Could you check a few things on this drawing? It's one solid part, dimensions in mm from its lowest x, y, z. Give positions to 0.01 mm unless a question says otherwise; leave off trailing zeros. Order: outer loops, then holes, each group sorted by start corner. A loop starts at its lowest first (then second) coordinate and runs counter-clockwise, first axis right, second up. Notation, with made-up numbers: (38.25, -13) -> (84.25, -13) arc R25 cw to (84.25, 2) -> close; hole circle Ø9 at (34, 18). An arc over 180 degrees is marked (long way). Write each question's results on one line, items separated by ' | '. Start each with the question number.
Q1. I'm going to push flat-ended pins straight in: pin 1 (1.5 mm diameter, centred on x = 97, z = 1.5, fed in from -Y); pin 2 (1.5 mm diameter, centred on x = 50.5, z = 2, fed in from +Y). Where does each tip first touch, or does it pass through?
Q2. Imagine slicing it at C-C, the plane x = 30. Please give me the cut outline in (y, z).
Q3. I need wall thicknesses on line 1 along X through (y, z) = (71.5, 2.2); line 2 along X through (y, z) = (10, 0.65); line 3 along Y through (x, z) = (19, 1.1). Which ranges of each line are inside material? Lowest first, please. Write a range as [from, to].
Q4. Imagine slicing it at B-B, the plane z = 1.45. State how many separate pieces and enclosed holes the cut face has, then the cut area to 3 significant figures.
Q5. Imagine slicing it at A-A, the plane y = 25.4. Please give me the cut outline in (x, z) (1 decimal).
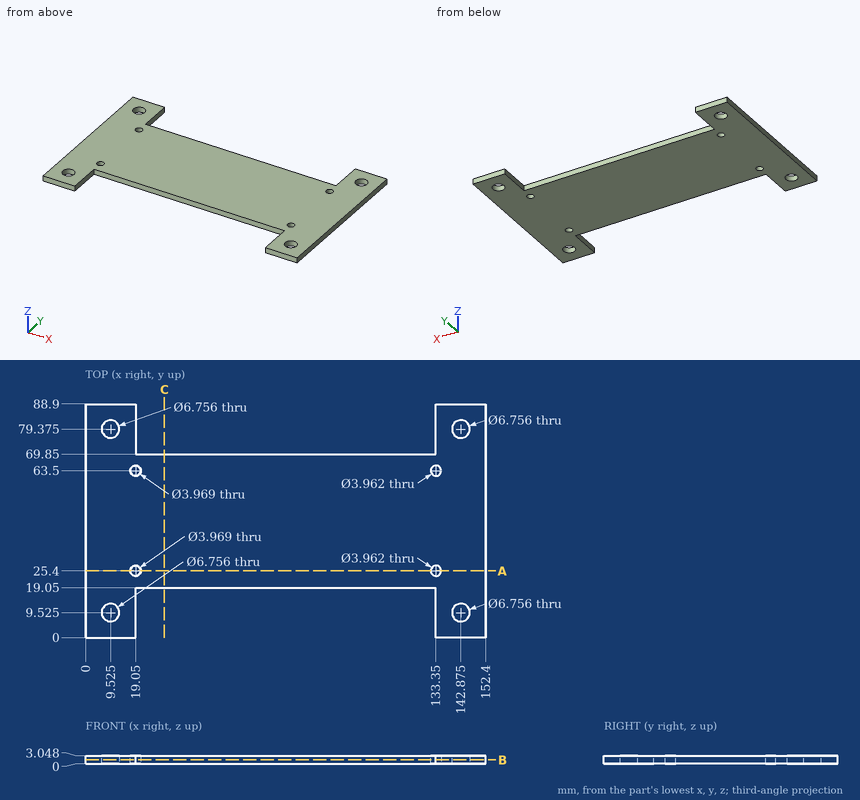
Geometry check:
1) pin 1: y = 19.05 | pin 2: y = 69.85
2) outline: (19.05, 0) -> (69.85, 0) -> (69.85, 3.05) -> (19.05, 3.05) -> close
3) line 1: [0, 19.05], [133.35, 152.4] | line 2: [0, 6.18], [12.87, 19.05], [133.35, 139.53], [146.22, 152.4] | line 3: [0, 23.42], [27.38, 61.52], [65.48, 88.9]
4) separate pieces: 1 | enclosed holes: 8 | area: 9,000 mm²
5) outline: (0, 0) -> (17.1, 0) -> (17.1, 3) -> (0, 3) -> close; (21, 0) -> (131.4, 0) -> (131.4, 3) -> (21, 3) -> close; (135.3, 0) -> (152.4, 0) -> (152.4, 3) -> (135.3, 3) -> close
